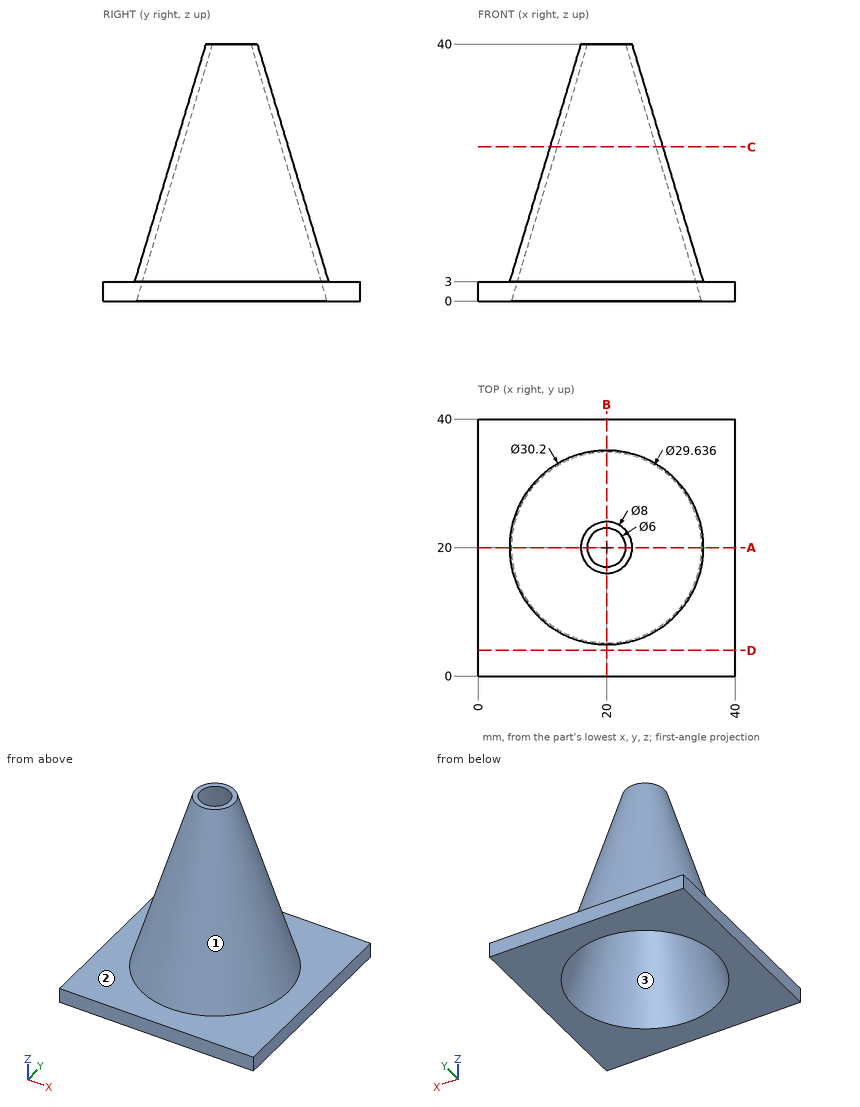
Job drawing, mm, ordinate dimensions from the low corner. One solid piece. Round coordinates to 2 decimals unless told otherwise and drop trailing zeros. Loops run counter-clockwise (first coordinate to the right, second up) from the corner with the lowest first, then second, coordinate; pieces in that order, holes last.
(1) Drop flat-ended pins along their axis: pin 1 (1 mm diameter, centred on x = 10.5, z = 10.5, fed in from +Y) (1 decimal); pin 2 (4 mm diameter, centred on y = 27.5, z = 33, fed in from -X); pin 3 (3 mm diameter, centred on y = 23, z = 21.5, fed in from +X) (1 decimal). Give the stop position or say it passes through.
(2) Cut at D-D (y = 4). Give the cut face in (x, z).
(3) Wall check: line 1 along Z through (x, y) = (34, 32); line 2 along X through (y, z) = (14, 17); line 3 along X through (y, z) = (23.5, 34) (1 decimal). Give the ranges that are in metal, low to high.
(4) Cut at C-C (z = 24). Give the cut face in (x, y) (1 decimal).
(5) Two-plate mould, pull along Y, no slides. Class the marked faces 1, 2 and 3: +Y half, -Y half, draft (parallel to the pull), parting line (faces both ways), or undercut.
(6) Cut at A-A (y = 20). Give the cut face in (x, z), plus the area to 3 significant figures.
Findings below:
1. pin 1: stops at y = 29.2
1. pin 2: stops at x = 17.14
1. pin 3: stops at x = 29.7
2. outline: (0, 0) - (40, 0) - (40, 3) - (0, 3) - close
3. line 1: z = 0 to 3
3. line 2: x = 10.9 to 12.26, 27.74 to 29.1
3. line 3: x = 15.4 to 16.8, 23.2 to 24.6
4. outline: circle Ø17.6 at (20, 20); hole circle Ø15.5 at (20, 20)
5. face 1: parting line
5. face 2: draft
5. face 3: undercut
6. outline: (0, 0) - (5.18, 0) - (17, 40) - (16, 40) - (4.9, 3) - (0, 3) - close; (23, 40) - (34.82, 0) - (40, 0) - (40, 3) - (35.1, 3) - (24, 40) - close
6. area: 114 mm2
